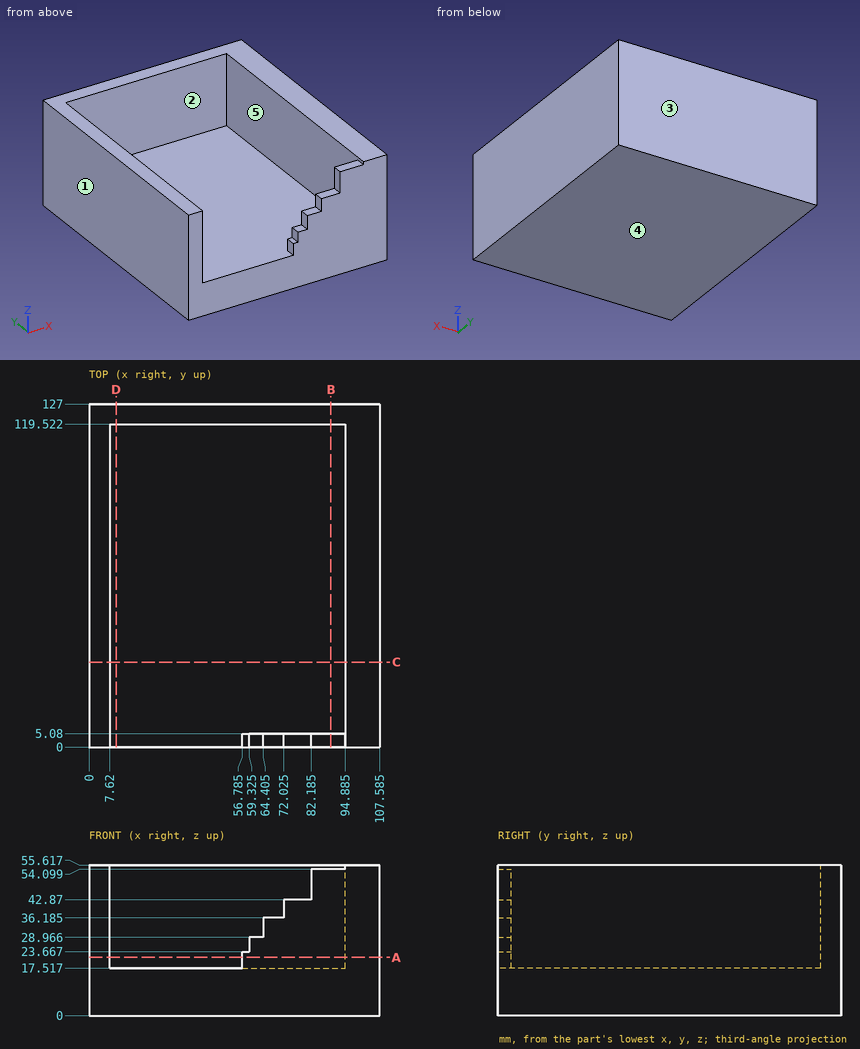
Verification items for this drawing (mm, ordinates from the low corner). A direction names the side the tool comes from. Round coordinates to 2 decimals unless told otherwise and drop trailing zeros. Write each loop counter-clockwise with the first axis right and the second up, starting at its lowest first coordinate (ties: lowest second). Pieces come first, ordered by that corner, then holes. Notation, with made-up numbers: (1.5, 68.5) - (23.5, 68.5) arc R14 cw to (23.5, 90.5) - close; hole circle Ø4 at (52, -16.75). An arc over 180 degrees is marked (long way). One line per item, written item: value.
1. Mould release check, pull along Y, two halves, no side actions. Record for the marked faces 1, 2 and 3: released by +Y, released by -Y, zero draft, split by the parting line, or undercut.
The answers:
face 1: zero draft
face 2: undercut
face 3: released by +Y
2. Scan lines: L1, parallel to X at y = 119, z = 28 (1 decimal); L2, parallel to Y at x = 64.5, z = 24; L3, parallel to Z at x = 39, y = 113. Record each from-to range of solid material in increasing order.
The answers:
L1: x = 0 to 7.6, 94.9 to 107.6
L2: y = 0 to 5.08, 119.52 to 127
L3: z = 0 to 17.52
3. Set-up check for the marked faces 4 and 5: record each of +Z, -Z, +X, -X, +Y, -Y from which the full face is reachable in a straight line by a thin tool's end or side.
The answers:
face 4: -Z, +X, -X, +Y, -Y
face 5: +Z
4. Cross-section at C-C on y = 31.5. Record the boundary of the cut face in (x, z) (1 decimal).
The answers:
outline: (0, 0) - (107.6, 0) - (107.6, 55.6) - (94.9, 55.6) - (94.9, 17.5) - (7.6, 17.5) - (7.6, 55.6) - (0, 55.6) - close
5. Depth check by flat-ended pin: pin 1 Ø5.5 at (x, y) = (61.5, 2.5) entering from +Z; pin 2 Ø5.5 at (x, y) = (89.5, 2) entering from +Z; pin 3 Ø0.8 at (x, y) = (58, 2) entering from +Z. Enter the tip coordinate at first touch or a pass-through.
The answers:
pin 1: stops at z = 28.97
pin 2: stops at z = 54.1
pin 3: stops at z = 23.67
6. Cross-section at D-D on x = 10. Record the boundary of the cut face in (y, z).
The answers:
outline: (0, 0) - (127, 0) - (127, 55.62) - (119.52, 55.62) - (119.52, 17.52) - (0, 17.52) - close
7. Cross-section at A-A on z = 21.5. Record the boundary of the cut face in (x, y) (1 decimal).
The answers:
outline: (0, 0) - (7.6, 0) - (7.6, 119.5) - (94.9, 119.5) - (94.9, 5.1) - (56.8, 5.1) - (56.8, 0) - (107.6, 0) - (107.6, 127) - (0, 127) - close
8. Cross-section at B-B on x = 89.5. Record the boundary of the cut face in (y, z).
The answers:
outline: (0, 0) - (127, 0) - (127, 55.62) - (119.52, 55.62) - (119.52, 17.52) - (5.08, 17.52) - (5.08, 54.1) - (0, 54.1) - close
